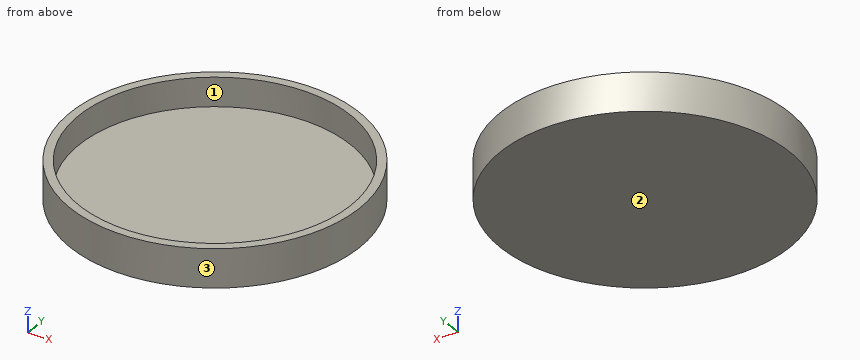
Autodesk Fusion 360 part; units mm, degrees
sketch "Sketch1" plane through (0, 0, 0) normal (0, 0, 1) x (1, 0, 0) in component "Component"
  line L0 (3.8891, 2.4749) -> (5.2486, 3.8344)
  circle A0 centre (0, 0) radius 6.5
  line L1 (-2.4749, 3.8891) -> (-3.8344, 5.2486)
  circle A1 centre (0, 0) radius 7.05
  line L2 (3.182, 3.182) -> (2.4749, 3.8891)
  line L3 (-3.182, 3.182) -> (-3.8891, 2.4749)
  line L4 (-3.182, -3.182) -> (-2.4749, -3.8891)
  line L5 (-3.8891, -2.4749) -> (-5.2486, -3.8344)
  line L6 (2.4749, -3.8891) -> (3.8344, -5.2486)
  line L7 (-2.4749, -3.8891) -> (-3.8344, -5.2486)
  line L8 (3.182, -3.182) -> (2.4749, -3.8891)
  line L9 (-3.182, -3.182) -> (-3.8891, -2.4749)
  circle A2 centre (0, 0) radius 7.5
  line L10 (3.182, 3.182) -> (3.8891, 2.4749)
  line L11 (-3.8891, 2.4749) -> (-5.2486, 3.8344)
  line L12 (-3.182, 3.182) -> (-2.4749, 3.8891)
  line L13 (3.8891, -2.4749) -> (5.2486, -3.8344)
  line L14 (3.182, -3.182) -> (3.8891, -2.4749)
  line L15 (2.4749, 3.8891) -> (3.8344, 5.2486)
  circle A3 centre (0, 0) radius 1.5
  dimension "d1" = 15
  dimension "d2" = 14.1
  dimension "d3" = 13
  dimension "d8" = 3
extrude "Extrude1" add sketch "Sketch1" along normal blind 2 contours A2 in component "Component"
extrude "Extrude2" add sketch "Sketch1" along normal blind 0.5 contours L0 A0 L2 L10 L15 | L0 A0 L1 L2 L3 L4 L5 L6 L7 L8 L9 L10 L11 L12 L13 L14 L15 | A0 L6 L8 L13 L14 | A0 L1 L3 L11 L12 | A0 L4 L5 L7 L9 | A1 | A3 in component "Component"
extrude "Extrude3" add sketch "Sketch1" along normal blind 30.5 contours A3 in component "Component"
extrude "Extrude4" cut 1 faces at (0.567, -0.5383, 30.5) along direction (0, 0, -1) blind 30 in component "Component"
extrude "Extrude5" add sketch "Sketch1" along normal blind 30.5 contours A3 in component "Component"
extrude "Extrude6" cut 1 faces at (0.567, -0.5383, 30.5) along direction (0, 0, -1) blind 30 in component "Component"
component "Component" placed x (1, 0, 0) y (0, 1, 0) z (0, 0, 1) at (0, 0, 0)
The listing builds one solid part. Answer for the finished solid, in the listing's coordinates (mm). Face numbers are marked on the shaded views. Give positions to 0.01 mm unless a question says otherwise; leave off trailing zeros. Loops run counter-clockwise (first coordinate to the right, second up) from the corner with the lowest first, then second, coordinate; pieces in that order, holes last. Notation, with made-up numbers: M 88.25,23 L 113.25,23 A21 cw 113.25,41 Z; hole C 88,-8.75 d6. An arc over 180 degrees is marked long. Answer as CSV lines item,"result".
Item 1: The part is cut by section A-A (y = 0). Give the vertices of the cut face in (x, z), and give its area (3 significant figures).
Values follow:
outline,"M -7.5,0 L 7.5,0 L 7.5,2 L 7.05,2 L 7.05,0.5 L -7.05,0.5 L -7.05,2 L -7.5,2 Z"
area,"8.85 mm^2"
Item 2: Straight lines are drawn through the part: line 1 along Y through (x, z) = (0, 1.5); line 2 along X through (y, z) = (-2, 0.8). For each, find the intervals that lie inside material, in ascending order. Write a range as [from, to].
Values follow:
line 1,"y = [-7.5, -7.05], [7.05, 7.5]"
line 2,"x = [-7.23, -6.76], [6.76, 7.23]"
Item 3: The mould has two halves that part along Y. Classify the marked faces 1, 2 and 3: released by +Y, released by -Y, zero draft, split by the parting line, or undercut.
Values follow:
face 1,"undercut"
face 2,"zero draft"
face 3,"split by the parting line"
Item 4: Given pin 1 Ø8 at (x, y) = (1, -2) entering from +Z, flat-ended and moving along its own axis, determine where the tip first touches the part or whether it passes through.
Values follow:
pin 1,"stops at z = 0.5"
Item 5: The part is cut by section B-B (z = 1.6). Give the vertices of the cut face in (x, y).
Values follow:
outline,"C 0,0 d15; hole C 0,0 d14.1"
